CAD build for the part. Positions are in the model's coordinates, mm. A direction names the side the tool comes from. Coordinates: 2 decimals unless noted, no trailing zeros. Loops run counter-clockwise (first coordinate to the right, second up) from the corner with the lowest first, then second, coordinate; pieces in that order, holes last. Notation, with made-up numbers: (-36, -36.5) - (-23, -36.5) arc R21 cw to (-23, -30.5) - close; hole circle Ø11 at (76.25, 28). An arc over 180 degrees is marked (long way). Put each result on its own line as item: value.
```python
from build123d import *
from OCP.BRepFilletAPI import BRepFilletAPI_MakeChamfer

# Parameters (mm, degrees)
SKETCH_1_R          = 25
EXTRUDE_1_DEPTH     = 50
CHAMFER_1_SIZE      = 5
CHAMFER_1_SIZE2     = 3.372542584
CUT_EXTRUDE_START   = -20
SKETCH_2_R          = 25
SKETCH_2_R_2        = 24.5
CUT_EXTRUDE_1_DEPTH = 20


with BuildPart() as part:
    # 草图1 → 凸台-拉伸1 (new, symmetric)
    with BuildSketch(Plane.XY):
        Circle(SKETCH_1_R)
    extrude(amount=EXTRUDE_1_DEPTH, both=True)

    # 倒角1: one chamfer whose edges measure the first distance from different faces: ONE call of the kernel's chamfer builder (chamfer() names one face for all edges)
    chamfer_1_edges_1 = [part.edges().sort_by_distance(p)[0] for p in [
        (-25, 0, -50),
    ]]
    chamfer_1_side_1 = [part.faces().sort_by_distance(p)[0] for p in [
        (0, 0, -50),
    ]]
    chamfer_1_edges_2 = [part.edges().sort_by_distance(p)[0] for p in [
        (-25, 0, 50),
    ]]
    chamfer_1_side_2 = [part.faces().sort_by_distance(p)[0] for p in [
        (-25, 0, 0),
    ]]
    chamfer_1 = BRepFilletAPI_MakeChamfer(part.part.solid().wrapped)
    for e in chamfer_1_edges_1:
        chamfer_1.Add(CHAMFER_1_SIZE, CHAMFER_1_SIZE2, e.wrapped, chamfer_1_side_1[0].wrapped)  # the first distance lies on this face
    for e in chamfer_1_edges_2:
        chamfer_1.Add(CHAMFER_1_SIZE, CHAMFER_1_SIZE2, e.wrapped, chamfer_1_side_2[0].wrapped)  # the first distance lies on this face
    add(Compound.cast(chamfer_1.Shape()), mode=Mode.REPLACE)

    # 草图2 → 切除-拉伸1 (cut)
    with BuildSketch(Plane(origin=(0, 0, 0), x_dir=(-1, 0, 0), z_dir=(0, 0, -1)).offset(CUT_EXTRUDE_START)):
        Circle(SKETCH_2_R)
        Circle(SKETCH_2_R_2, mode=Mode.SUBTRACT)
    extrude(amount=CUT_EXTRUDE_1_DEPTH, mode=Mode.SUBTRACT)


solid = part.part
```
Q1. Tool access for faces 4 (the flat face through (-18, -17, 20)), 5 (the conical face through (19.37, 6.1, -49.79)): list every direction of +Z, -Z, +X, -X, +Y, -Y with a clear straight run to the whole face (end or side of a thin tool).
Determined:
face 4: none
face 5: -Z
Q2. Wall check: L1, parallel to Y at x = -0.5, z = -23 (3 decimals); L2, parallel to Y at x = -19, z = -38; L3, parallel to Z at x = 18, y = -13.5. Give the ranges that are in metal, low to high. Write a range as from..to.
Determined:
L1: -24.995..24.995
L2: -16.25..16.25
L3: -48.31..48.71
Q3. Pin check, flat tips, straight feed: pin 1 Ø2 at (x, z) = (-9.5, -33) entering from -Y; pin 2 Ø1.5 at (y, z) = (16.5, 32) entering from +X; pin 3 Ø5 at (x, z) = (-18.5, 23.5) entering from +Y. Stop position of each tip, or through.
Determined:
pin 1: y = -23.51
pin 2: x = 19.41
pin 3: y = 19.21
Q4. Slice it at A-A, the plane z = -19. Give the cut face in (x, y), then the cut area to 3 significant figures.
Determined:
outline: circle Ø50 at (0, 0)
area: 1,960 mm2
Q5. Slice it at B-B, the plane z = 18. Give the cut face in (x, y).
Determined:
outline: circle Ø49 at (0, 0)
Q6. Mould opens along Z. For faces 1 (the flat face through (0, 0, 50)), 2 (the flat face through (-18, -17, 0)), 3 (the cylindrical face through (23.846, 7.509, 32.675)) say: +Z half, -Z half, draft (parallel to the pull), parting line (faces both ways), or undercut.
Determined:
face 1: +Z half
face 2: undercut
face 3: draft
